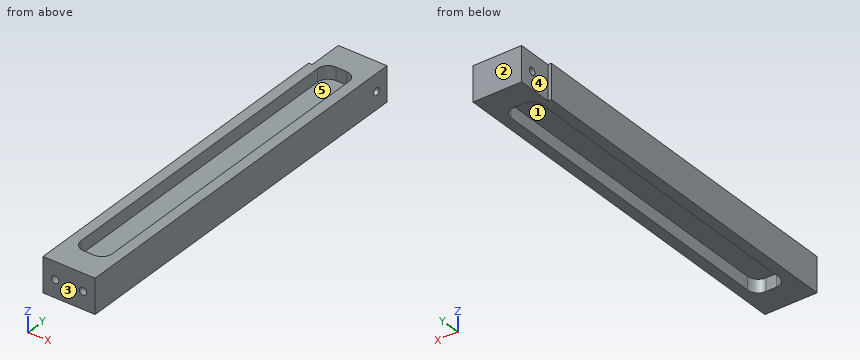
```python
from build123d import *

# Parameters (mm, degrees)
SKETCH_1_W             = 30
SKETCH_1_H             = 20
EXTRUDE_1_DEPTH        = 222
CUT_EXTRUDE_1_DEPTH    = 7.5
HOLE_WIZARD_M5_1_D     = 4.2
HOLE_WIZARD_M5_1_DEPTH = 14
HOLE_WIZARD_M5_1_TIP   = 1.2618073
HOLE_WIZARD_M5_2_D     = 4.2
CUT_EXTRUDE_2_DEPTH    = 224.403222895


with BuildPart() as part:
    # 草图1 → 凸台-拉伸1 (new body)
    with BuildSketch(Plane(origin=(0, 0, 0), x_dir=(1, 0, 0), z_dir=(0, 1, 0))):
        Rectangle(SKETCH_1_W, SKETCH_1_H)
    extrude(amount=EXTRUDE_1_DEPTH)

    # 草图2 → 切除-拉伸1 (cut)
    with BuildSketch(Plane.XY.offset(-10)):
        with BuildLine():
            Line((-3, 15), (3, 15))
            ThreePointArc((3, 15), (7.242640687, 16.757359313), (9, 21))
            Line((9, 21), (9, 201))
            ThreePointArc((9, 201), (7.242640687, 205.242640687), (3, 207))
            Line((3, 207), (-3, 207))
            ThreePointArc((-3, 207), (-7.242640687, 205.242640687), (-9, 201))
            Line((-9, 201), (-9, 21))
            ThreePointArc((-9, 21), (-7.242640687, 16.757359313), (-3, 15))
        make_face()
    cut_extrude_1 = extrude(amount=CUT_EXTRUDE_1_DEPTH, mode=Mode.SUBTRACT)

    # 镜向1: 切除-拉伸1 across plane
    add(cut_extrude_1.mirror(Plane.XY), mode=Mode.SUBTRACT)

    # M5 螺纹孔1
    with Locations(Plane(origin=(0, 0, 0), x_dir=(-1, 0, 0), z_dir=(0, -1, 0))):
        with Locations((8, 0), (-8, 0)):
            Hole(HOLE_WIZARD_M5_1_D / 2, depth=HOLE_WIZARD_M5_1_DEPTH)
            with Locations((0, 0, -(HOLE_WIZARD_M5_1_DEPTH + HOLE_WIZARD_M5_1_TIP / 2))):  # 118° drill point
                Cone(0, HOLE_WIZARD_M5_1_D / 2, HOLE_WIZARD_M5_1_TIP, mode=Mode.SUBTRACT)

    # M5 螺纹孔2 (through all)
    with Locations(Plane(origin=(15, 0, 0), x_dir=(0, 0, -1), z_dir=(1, 0, 0))):
        with Locations((0, 214)):
            Hole(HOLE_WIZARD_M5_2_D / 2)

    # 草图7 → 切除-拉伸2 (cut, through all)
    with BuildSketch(Plane(origin=(0, 0, 10), x_dir=(-1, 0, 0), z_dir=(0, 0, -1))):
        Polygon((13, 679.517597419), (13, 222), (13, 202), (15, 202), (472.517597419, 202), (1131.852642703, 836.481446423), (672.335045283, 1313.999043842), align=None)
    extrude(amount=CUT_EXTRUDE_2_DEPTH, mode=Mode.SUBTRACT)


solid = part.part
```
Part model, mm, in its own coordinate system. Face numbers are marked on the shaded views. A direction names the side the tool comes from. Give positions to 0.01 mm unless a question says otherwise; leave off trailing zeros. Write each loop counter-clockwise with the first axis right and the second up, starting at its lowest first coordinate (ties: lowest second). Pieces come first, ordered by that corner, then holes. Notation, with made-up numbers: (-24.75, 70) -> (7.25, 70) arc R11 ccw to (7.25, 91) -> close; hole circle Ø8 at (7, -2.75). An arc over 180 degrees is marked (long way). Put each result on its own line as item: value. Start each with the question number.
Item 1: Cut at A-A (z = 7.75). List the corners of the cut face in (x, y), then the cut area to 3 significant figures.
Item 2: Cut at C-C (y = 91.5). List the corners of the cut face in (x, z).
Item 3: Wall check: L1, parallel to Y at x = 0.25, z = -7; L2, parallel to Z at x = -8, y = 8; L3, parallel to X at y = 50, z = -7.5. Give the ranges that are in metal, low to high. Write a range as [from, to].
Item 4: Pin check, flat tips, straight feed: pin 1 Ø14.5 at (x, y) = (1, 114.5) entering from +Z; pin 2 Ø3.5 at (x, z) = (8, 0) entering from -Y; pin 3 Ø1 at (x, y) = (-8, 101.5) entering from -Z. Stop position of each tip, or through.
Item 5: Which spindle directions (+Z, -Z, +X, -X, +Y, -Y) get a long thin tool onto all of the face, cutting with end or side? Do the marked faces 1 and 2. Say none if no direction does.
Item 6: Cut at B-B (y = 214). List the corners of the cut face in (x, z), then the cut area to 3 significant figures.
Item 7: Cut at D-D (y = 17.5). List the corners of the cut face in (x, z).
Item 8: Pull direction Y, two halves, no side cores. Call the marked faces 3, 4 and 5: pulls with the +Y half, pulls with the -Y half, needs draft (parallel to the pull), parting line crosses it, or undercut.
Answer list:
1. outline: (-15, 0) -> (15, 0) -> (15, 222) -> (-13, 222) -> (-13, 202) -> (-15, 202) -> close; hole (-9, 21) arc R6 ccw to (-3, 15) -> (3, 15) arc R6 ccw to (9, 21) -> (9, 201) arc R6 ccw to (3, 207) -> (-3, 207) arc R6 ccw to (-9, 201) -> close
1. area: 3,190 mm2
2. outline: (-15, -10) -> (-9, -10) -> (-9, -2.5) -> (9, -2.5) -> (9, -10) -> (15, -10) -> (15, 10) -> (9, 10) -> (9, 2.5) -> (-9, 2.5) -> (-9, 10) -> (-15, 10) -> close
3. L1: y = [0, 15], [207, 222]
3. L2: z = [-10, -2.1], [2.1, 10]
3. L3: x = [-15, -9], [9, 15]
4. pin 1: stops at z = 2.5
4. pin 2: stops at y = 14.21
4. pin 3: stops at z = -2.5
5. face 1: -Z
5. face 2: +Z, -Z, +X, -X, +Y
6. outline: (-13, -10) -> (15, -10) -> (15, -2.1) -> (-13, -2.1) -> close; (-13, 2.1) -> (15, 2.1) -> (15, 10) -> (-13, 10) -> close
6. area: 442 mm2
7. outline: (-15, -10) -> (-7.87, -10) -> (-7.87, -2.5) -> (7.87, -2.5) -> (7.87, -10) -> (15, -10) -> (15, 10) -> (7.87, 10) -> (7.87, 2.5) -> (-7.87, 2.5) -> (-7.87, 10) -> (-15, 10) -> close
8. face 3: pulls with the -Y half
8. face 4: needs draft
8. face 5: undercut
